Source: CAD feature listing. Evaluate the final solid. Frame: model axes, mm. Coordinates: 2 decimals unless noted, no trailing zeros. Write each loop counter-clockwise with the first axis right and the second up, starting at its lowest first coordinate (ties: lowest second). Pieces come first, ordered by that corner, then holes. Notation, with made-up numbers: M -14,-20.5 L -2,-20.5 A24 ccw -2,5.5 Z; hole C -33.5,40 d10. An arc over 180 degrees is marked long. Write item = value, one per line. Start each with the question number.
1. Section query C-C (x = 4). Output: boundary loops of the cut face in (y, z) (3 decimals), then the cut area to 3 significant figures.
2. Section query D-D (y = 8). Output: boundary loops of the cut face in (x, z) (3 decimals).
3. Line query: line 1 along Y through (x, z) = (0, 1.2); line 2 along X through (y, z) = (-0.5, 2.4); line 3 along X through (y, z) = (-12, 2.65). Output: solid intervals per line, ascending.
4. Section query A-A (y = 0). Output: boundary loops of the cut face in (x, z) (3 decimals).
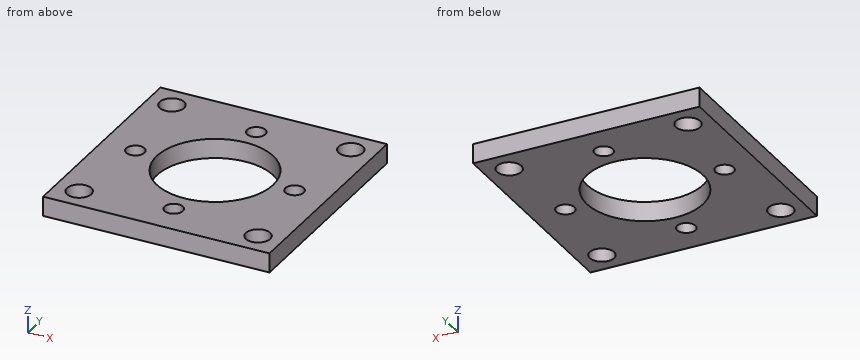
```python
from build123d import *

# Parameters (mm, degrees)
SKETCH1_W           = 37
SKETCH1_H           = 37
BOSS_EXTRUDE1_DEPTH = 3.175
SKETCH2_R           = 9.5
CUT_EXTRUDE1_DEPTH  = 27.354897552
SKETCH3_R           = 1.5
CUT_EXTRUDE2_DEPTH  = 27.354897552
SKETCH4_R           = 2
CUT_EXTRUDE3_DEPTH  = 27.354897552


with BuildPart() as part:
    # Sketch1 → Boss-Extrude1 (new body)
    with BuildSketch(Plane.XY):
        Rectangle(SKETCH1_W, SKETCH1_H)
    extrude(amount=BOSS_EXTRUDE1_DEPTH)

    # Sketch2 → Cut-Extrude1 (cut, through all)
    with BuildSketch(Plane.XY.offset(3.175)):
        Circle(SKETCH2_R)
    extrude(amount=-CUT_EXTRUDE1_DEPTH, mode=Mode.SUBTRACT)

    # Sketch3 → Cut-Extrude2 (cut, through all)
    with BuildSketch(Plane.XY.offset(3.175)):
        with Locations((-13, 0)):
            Circle(SKETCH3_R)
        with Locations((0, 13)):
            Circle(SKETCH3_R)
        with Locations((13, 0)):
            Circle(SKETCH3_R)
        with Locations((0, -13)):
            Circle(SKETCH3_R)
    extrude(amount=-CUT_EXTRUDE2_DEPTH, mode=Mode.SUBTRACT)

    # Sketch4 → Cut-Extrude3 (cut, through all)
    with BuildSketch(Plane.XY.offset(3.175)):
        with Locations((-14.610912703, 14.610912703)):
            Circle(SKETCH4_R)
        with Locations((14.610912703, 14.610912703)):
            Circle(SKETCH4_R)
        with Locations((14.610912703, -14.610912703)):
            Circle(SKETCH4_R)
        with Locations((-14.610912703, -14.610912703)):
            Circle(SKETCH4_R)
    extrude(amount=-CUT_EXTRUDE3_DEPTH, mode=Mode.SUBTRACT)


solid = part.part
```
Results are:
q1.outline = M -18.5,0 L -8.617,0 L -8.617,3.175 L -18.5,3.175 Z; M 8.617,0 L 18.5,0 L 18.5,3.175 L 8.617,3.175 Z
q1.area = 62.8 mm^2
q2.outline = M -18.5,0 L -5.123,0 L -5.123,3.175 L -18.5,3.175 Z; M 5.123,0 L 18.5,0 L 18.5,3.175 L 5.123,3.175 Z
q3.line_1 = -18.5 to -14.5, -11.5 to -9.5, 9.5 to 11.5, 14.5 to 18.5
q3.line_2 = -18.5 to -14.41, -11.59 to -9.49, 9.49 to 11.59, 14.41 to 18.5
q3.line_3 = -18.5 to -1.12, 1.12 to 18.5
q4.outline = M -18.5,0 L -14.5,0 L -14.5,3.175 L -18.5,3.175 Z; M -11.5,0 L -9.5,0 L -9.5,3.175 L -11.5,3.175 Z; M 9.5,0 L 11.5,0 L 11.5,3.175 L 9.5,3.175 Z; M 14.5,0 L 18.5,0 L 18.5,3.175 L 14.5,3.175 Z
